Verification items for the finished model (mm, model axes). A direction names the side the tool comes from. Round coordinates to 2 decimals unless told otherwise and drop trailing zeros. Order: outer loops, then holes, each group sorted by start corner. A loop starts at its lowest first (then second) coordinate and runs counter-clockwise, first axis right, second up. Notation, with made-up numbers: (48.25, 81) -> (54.25, 81) arc R14 cw to (54.25, 94) -> close; hole circle Ø7 at (-29.5, -6.5). An arc over 180 degrees is marked (long way). Return JSON: item names as keys, results as strings. Group by question number.
1) Section check C-C on x = -38. Enter the section's corners in (y, z), plus the area to 3 significant figures.
2) Section check A-A on x = -8. Enter the section's corners in (y, z).
3) Depth check by flat-ended pin: pin 1 (1 mm diameter, centred on y = -3.5, z = 4, fed in from +X); pin 2 (2.5 mm diameter, centred on x = -38, z = -4, fed in from +Y); pin 3 (2 mm diameter, centred on y = -6, z = 19.5, fed in from +X); pin 4 (1 mm diameter, centred on x = -30, y = -2.5, fed in from +Z). Enter the tip coordinate at first touch or a pass-through.
4) Section check D-D on z = -4. Enter the section's corners in (x, y), plus the area to 3 significant figures.
5) Tool access check on faces 1 (the flat face through (-30, -4, 0)), 2 (the cylindrical face through (-0.86, -4.56, -7.1)). Record the directions out of +Z, -Z, +X, -X, +Y, -Y that give a thin tool (end or side, any length) a straight path to the whole face; none if there is none.
6) Section check B-B on z = 26. Enter the section's corners in (x, y).
7) Scan lines: L1, parallel to Z at x = -38, y = -4.75; L2, parallel to X at y = -4, z = 26; L3, parallel to Z at x = -8, y = -7. Record each from-to range of solid material in increasing order.
8) Draft check along X on faces 3 (the cylindrical face through (-6.69, -4.56, -3)), 4 (the cylindrical face through (-41.14, -4.56, -7.1)), 5 (the cylindrical face through (-0.86, -4.56, -0.9)). Enter one of: pulls with the +X half, pulls with the -X half, needs draft (parallel to the pull), parting line crosses it, or undercut.
```python
from build123d import *

# Parameters (mm, degrees)
F1_DEPTH = 9
F2_R     = 3
F3_D     = 3.3


with BuildPart() as f1:
    # F0 (on Front) → F1 (new body)
    with BuildSketch(Plane.XZ):
        with BuildLine():
            Line((0, -8), (0, 0))
            Line((0, 0), (-13, 0))
            ThreePointArc((-13, 0), (-21, -0.9371725321), (-29, 0))
            Line((-29, 0), (-34, 0))
            Line((-34, 0), (-34, 5))
            ThreePointArc((-34, 5), (-34.9498381987, 13), (-34, 21))
            Line((-34, 21), (-34, 34))
            Line((-34, 34), (-42, 34))
            Line((-42, 34), (-42, 0))
            Line((-42, 0), (-42, -8))
            Line((-42, -8), (0, -8))
        make_face()
    extrude(amount=F1_DEPTH)

    # F2
    f2_edges = [f1.edges().sort_by_distance(p)[0] for p in [
        (-34, -4.5, 34),
        (-42, -4.5, 34),
        (0, -4.5, 0),
        (0, -4.5, -8),
        (-34, -4.5, 0),
        (-42, -4.5, -8),
    ]]
    fillet(f2_edges, radius=F2_R)

    # F3 (through all)
    with Locations(Plane(origin=(0, 0, 0), x_dir=(1, 0, 0), z_dir=(0, 1, 0))):
        with Locations((-38, -26), (-38, 4), (-8, 4)):
            Hole(F3_D / 2)


solid = f1.part
```
Check result:
{
 "1": {"outline": "(-9, -8) -> (0, -8) -> (0, -5.65) -> (-9, -5.65) -> close; (-9, -2.35) -> (0, -2.35) -> (0, 24.35) -> (-9, 24.35) -> close; (-9, 27.65) -> (0, 27.65) -> (0, 34) -> (-9, 34) -> close", "area": "319 mm^2"},
 "2": {"outline": "(-9, -8) -> (0, -8) -> (0, -5.65) -> (-9, -5.65) -> close; (-9, -2.35) -> (0, -2.35) -> (0, 0) -> (-9, 0) -> close"},
 "3": {"pin 1": "x = -34", "pin 2": "through", "pin 3": "x = -34.12", "pin 4": "z = 0"},
 "4": {"outline": "(-42, -9) -> (-39.65, -9) -> (-39.65, 0) -> (-42, 0) -> close; (-36.35, -9) -> (-9.65, -9) -> (-9.65, 0) -> (-36.35, 0) -> close; (-6.35, -9) -> (0, -9) -> (0, 0) -> (-6.35, 0) -> close", "area": "319 mm^2"},
 "5": {"face 1": "+Z, +X, +Y, -Y", "face 2": "-Z, +X, +Y, -Y"},
 "6": {"outline": "(-42, -9) -> (-39.65, -9) -> (-39.65, 0) -> (-42, 0) -> close; (-36.35, -9) -> (-34, -9) -> (-34, 0) -> (-36.35, 0) -> close"},
 "7": {"L1": "-8 to -5.65, -2.35 to 24.35, 27.65 to 34", "L2": "-42 to -39.65, -36.35 to -34", "L3": "-8 to -5.65, -2.35 to 0"},
 "8": {"face 3": "undercut", "face 4": "pulls with the -X half", "face 5": "pulls with the +X half"}
}
